Design review of the part shown in the three views and the two pictorial views. Dimensions are in mm from the part's minimum x, y and z. A direction names the side the tool comes from. Coordinates: 2 decimals unless noted, no trailing zeros. Loops run counter-clockwise (first coordinate to the right, second up) from the corner with the lowest first, then second, coordinate; pieces in that order, holes last. Notation, with made-up numbers: (69.25, -11) - (123.25, -11) arc R14 ccw to (123.25, -5) - close; hole circle Ø3 at (-38.5, -13.75). An arc over 180 degrees is marked (long way). One line per question, with ' | ' between items.
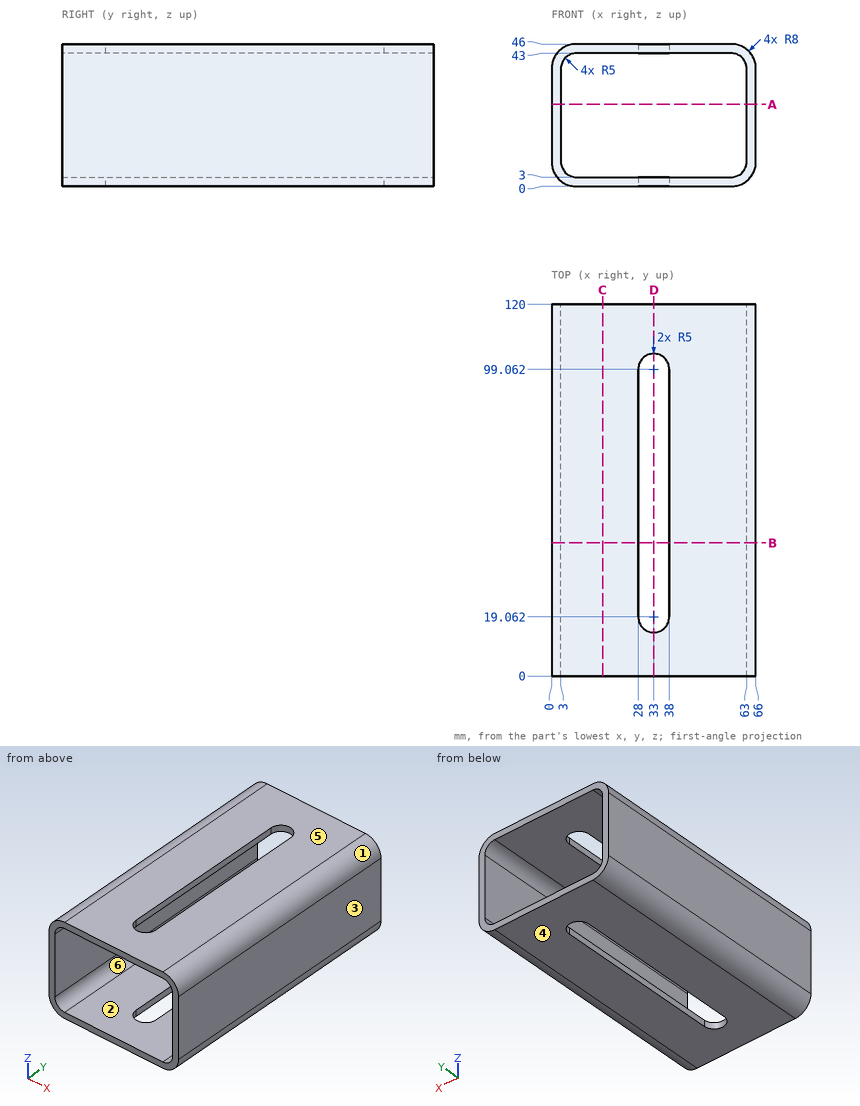
Q1. Take a section at A-A (z = 26.5). Give the boundary of the cut face in (x, y), plus the area to 3 significant figures.
Returned:
outline: (0, 0) - (3, 0) - (3, 120) - (0, 120) - close; (63, 0) - (66, 0) - (66, 120) - (63, 120) - close | area: 720 mm²
Q2. Take a section at D-D (x = 33). Give the boundary of the cut face in (y, z).
Returned:
outline: (0, 0) - (14.06, 0) - (14.06, 3) - (0, 3) - close; (0, 43) - (14.06, 43) - (14.06, 46) - (0, 46) - close; (104.06, 0) - (120, 0) - (120, 3) - (104.06, 3) - close; (104.06, 43) - (120, 43) - (120, 46) - (104.06, 46) - close
Q3. To check wall thickness, follow line 1 along X through (y, z) = (79.5, 35.5); line 2 along Z through (x, y) = (42, 48.5); line 3 along X through (y, z) = (59.5, 7). State the ranges of each line that lie inside material, in increasing order.
Returned:
line 1: x = 0 to 3, 63 to 66 | line 2: z = 0 to 3, 43 to 46 | line 3: x = 0.06 to 3.1, 62.9 to 65.94
Q4. Tool access review of the marked faces 1 and 2: name each direction out of +Z, -Z, +X, -X, +Y, -Y from which nothing blocks a thin tool from reaching the whole face with its end or side.
Returned:
face 1: +Z, +X, +Y, -Y | face 2: +Y, -Y
Q5. Draft analysis for pull direction Z (two halves, no side actions). For the marked faces 3, 4, 5 and 6, state which applies: +Z half, -Z half, draft (parallel to the pull), parting line (faces both ways), or undercut.
Returned:
face 3: draft | face 4: -Z half | face 5: +Z half | face 6: undercut
Q6. Take a section at C-C (x = 16.5). Give the boundary of the cut face in (y, z), plus the area to 3 significant figures.
Returned:
outline: (0, 0) - (120, 0) - (120, 3) - (0, 3) - close; (0, 43) - (120, 43) - (120, 46) - (0, 46) - close | area: 720 mm²
Q7. Take a section at B-B (y = 43). Give the boundary of the cut face in (x, z).
Returned:
outline: (0, 8) arc R8 ccw to (8, 0) - (28, 0) - (28, 3) - (8, 3) arc R5 cw to (3, 8) - (3, 38) arc R5 cw to (8, 43) - (28, 43) - (28, 46) - (8, 46) arc R8 ccw to (0, 38) - close; (38, 0) - (58, 0) arc R8 ccw to (66, 8) - (66, 38) arc R8 ccw to (58, 46) - (38, 46) - (38, 43) - (58, 43) arc R5 cw to (63, 38) - (63, 8) arc R5 cw to (58, 3) - (38, 3) - close
Q8. For pin 1 (2.5 mm diameter, centred on y = 49, z = 44.5, fed in from -X) (1 decimal); pin 2 (2.5 mm diameter, centred on y = 57.5, z = 44, fed in from +X); pin 3 (2.5 mm diameter, centred on y = 59.5, z = 1, fed in from -X); pin 4 (2 mm diameter, centred on x = 16.5, z = 4.5, fed in from +Y), all flat-tipped, find the tip position at first contact; note any pin that passes through.
Returned:
pin 1: stops at x = 2 | pin 2: stops at x = 64.44 | pin 3: stops at x = 2.44 | pin 4: passes through
